The model under review builds one solid part; all positions refer to its coordinate system, in mm. A direction names the side the tool comes from. Coordinates: 2 decimals unless noted, no trailing zeros. Order: outer loops, then holes, each group sorted by start corner. A loop starts at its lowest first (then second) coordinate and runs counter-clockwise, first axis right, second up. Notation, with made-up numbers: M 55,54.25 L 67,54.25 A9 ccw 67,59.25 Z; hole C 34,80 d5. An arc over 180 degrees is marked long. One line per item, written item: value.
Autodesk Inventor part; units mm, degrees
ref_plane "YZ Plane" through (0, 0, 0) normal (1, 0, 0) x (0, 1, 0)
ref_plane "XZ Plane" through (0, 0, 0) normal (0, 1, 0) x (-1, 0, 0)
ref_plane "XY Plane" through (0, 0, 0) normal (0, 0, 1) x (1, 0, 0)
sketch "Sketch1" plane through (0, 0, 0) normal (0, 1, 0) x (-1, 0, 0)
  line L0 (4, -12.0702) -> (4, 30.9298)
  line L1 (4, 30.9298) -> (-1, 30.9298)
  line L2 (-1, 30.9298) -> (-1, 25.9298)
  line L3 (-1, 25.9298) -> (-22, 25.9298)
  line L4 (4, -12.0702) -> (-1, -12.0702)
  line L5 (-1, -12.0702) -> (-1, -12.0702)
  line L6 (-22, -8.0702) -> (-22, -8.0702)
  line L7 (-22, -8.0702) -> (-22, 3.3216)
  line L8 (-22, 3.3216) -> (-22, 3.3216)
  line L9 (-22, 3.3216) -> (-22, 25.9298)
  line L10 (-1, -12.0702) -> (-5, -12.0702)
  line L11 (-5, -12.0702) -> (-5, -9.0702)
  line L12 (-5, -9.0702) -> (-16, -9.0702)
  arc A0 (-22, -11.4735) -> (-16, -11.4735) centre (-19, -15.0915) ccw
  line L13 (-16, -9.0702) -> (-16, -11.4735)
  line L14 (-22, -8.0702) -> (-22, -11.4735)
  point P0 (0, 0)
  dimension "d28" = 5
  dimension "d30" = 0
  dimension "d69" = 5
  dimension "d118" = 4
  dimension "d119" = 3
  dimension "d130" = 4.7
  dimension "d148" = 35
  dimension "d151" = 2.4033
extrude "Extrusion1" add sketch "Sketch1" along normal blind 13
sketch "Sketch5" plane through (0, 13, 0) normal (0, 1, 0) x (1, 0, 0)
  line L0 (-4, -30.9298) -> (1, -30.9298)
  line L1 (-1, -30.9298) -> (-4, -30.9298)
  line L2 (-4, -30.9298) -> (-4, -25.9298)
  line L3 (-4, -25.9298) -> (-1, -25.9298)
  line L4 (-1, -25.9298) -> (-1, -30.9298)
  line L5 (1, -30.9298) -> (1, -25.9298)
  line L6 (-4, 1.8702) -> (-1, 1.8702)
  line L7 (-1, 1.8702) -> (-1, -3.1298)
  line L8 (-1, -3.1298) -> (-4, -3.1298)
  line L9 (-4, -3.1298) -> (-4, 1.8702)
  line L10 (1, 12.0702) -> (1, 17.0702)
  line L11 (5, 12.0702) -> (-4, 12.0702)
  point P0 (0, 0)
  point P1 (-4, 12.0702)
  dimension "d60" = 5
  dimension "d61" = 3
  dimension "d62" = 2
  dimension "d63" = 2
  dimension "d64" = 3
  dimension "d65" = 5
  dimension "d149" = 22.8
extrude "Extrusion6" add sketch "Sketch5" along normal blind 12.3
sketch "Sketch6" plane through (-1, 13, 30.9298) normal (1, 0, 0) x (0, 0, -1)
  circle A0 centre (2.5, 6.15) radius 1
  line L0 (0, 12.3) -> (5, 12.3)
  line L1 (0, 0) -> (0, 12.3)
  circle A1 centre (30.3, 6.15) radius 1
  line L2 (27.8, 12.3) -> (32.8, 12.3)
  line L3 (27.8, 0) -> (27.8, 12.3)
  point P0 (30.9298, -13)
  dimension "d70" = 2
  dimension "d71" = 6.15
  dimension "d72" = 2.5
  dimension "d73" = 2
  dimension "d74" = 6.15
  dimension "d75" = 2.5
extrude "Extrusion7" cut sketch "Sketch6" against normal blind 12.3
thread "Thread6"
thread "Thread7"
sketch "Sketch10" plane through (0, 13, 0) normal (0, 1, 0) x (1, 0, 0)
  circle A0 centre (0.6, 10.2702) radius 1
  circle A1 centre (19.4, 10.2702) radius 1
  circle A2 centre (10, -8.7298) radius 1
  line L0 (1, -25.9298) -> (22, -25.9298)
  line L1 (-4, -3.1298) -> (-4, -25.9298)
  line L2 (5, 12.0702) -> (-4, 12.0702)
  line L3 (5, 9.0702) -> (5, 12.0702)
  line L4 (5, 12.0702) -> (1, 12.0702)
  point P0 (0, 0)
  point P1 (1, 17.0702)
  point P2 (-1, 17.0702)
  point P3 (-4, 12.0702)
  dimension "d108" = 2
  dimension "d109" = 2
  dimension "d110" = 2
  dimension "d111" = 9.4
  dimension "d112" = 9.4
  dimension "d113" = 19
  dimension "d117" = 19
  dimension "d121" = 14
  dimension "d150" = 1.8
extrude "Extrusion11" cut sketch "Sketch10" against normal blind 15
sketch "Sketch13" plane through (0, 13, 0) normal (0, 1, 0) x (1, 0, 0)
  point P0 (0, 0)
sketch "Sketch14" plane through (0, 0, 0) normal (0, -1, 0) x (1, 0, 0)
  circle A0 centre (19.4611, -14.5702) radius 2
  circle A1 centre (19.4, -10.2702) radius 1
  point P0 (0, 0)
  dimension "d131" = 4
  dimension "d132" = 4.3
extrude "Extrusion12" cut sketch "Sketch14" against normal blind 6 contours A0
sketch "Sketch15" plane through (0, 13, 0) normal (0, 1, 0) x (1, 0, 0)
  arc A0 (22, 11.4735) -> (16, 11.4735) centre (19, 15.0915) ccw
  line L0 (15.3998, 12.0702) -> (22.6002, 12.0702)
  arc A1 (22.6002, 12.0702) -> (15.3998, 12.0702) centre (19, 15.0915) ccw
  line L1 (1, -25.9298) -> (22, -25.9298)
  point P0 (0, 0)
  dimension "d135" = 22.8
extrude "Extrusion13" add sketch "Sketch15" along normal blind 12.5
sketch "Sketch16" plane through (0, 25.5, 0) normal (0, 1, 0) x (1, 0, 0)
  arc A0 (22, 11.4735) -> (16, 11.4735) centre (19, 15.0915) ccw
  circle A1 centre (19, 15.0915) radius 5
  point P0 (0, 0)
  dimension "d138" = 10
extrude "Extrusion14" add sketch "Sketch16" along normal mid plane 25
sketch "Sketch18" plane through (19, 38, -15.0915) normal (0, 1, 0) x (1, 0, 0)
  circle A0 centre (0, 0) radius 5
  point P0 (-19, -15.0915)
extrude "Extrusion16" add sketch "Sketch18" along normal blind 12.5
sketch "Sketch19" plane through (19, 50.5, -15.0915) normal (0, 1, 0) x (1, 0, 0)
  circle A0 centre (0, 0) radius 1.9
  point P0 (-19, -15.0915)
  dimension "d154" = 3.8
extrude "Extrusion17" add sketch "Sketch19" along normal blind 5
properties part number "4_2.(new).stl"
(1) Tool access review of faces 1 (the flat face through (19, 50.5, -13)), 2 (the cylindrical face through (19.94, 6.59, -11.11)), 3 (the flat face through (1, 6, 28)), 4 (the flat face through (0, 6, -12.07)): name each direction out of +Z, -Z, +X, -X, +Y, -Y from which nothing blocks a thin tool from reaching the whole face with its end or side.
Geometry results:
face 1: +Y
face 2: -Y
face 3: +Z, +X, +Y, -Y
face 4: -Z, -X, +Y, -Y
(2) For L1, parallel to X at y = 8, z = -11; L2, parallel to Z at x = 19.4, y = 5.25; L3, parallel to Z at x = 0.6, y = 6.75, list the stretches that pass through material, from the lowest coordinate up.
Geometry results:
L1: x = -4 to -0.08, 1.28 to 5, 16 to 18.72, 20.08 to 22
L2: z = -19.77 to -16.57, -12.57 to -11.27, -9.27 to 25.93
L3: z = -12.07 to -11.27, -9.27 to 30.93
(3) We need section A-A, the plane x = 10. State the section outline as (y, z) points.
Geometry results:
outline: M 0,-9.07 L 13,-9.07 L 13,7.73 L 0,7.73 Z; M 0,9.73 L 13,9.73 L 13,25.93 L 0,25.93 Z
(4) Mouldability with a two-part tool opening along Z and no side actions: class faces 5 (the flat face through (-3, 19, 25.93)), 6 (the cylindrical face through (17.92, 32.01, -10.21)), 7 (the flat face through (-1, 19, 30)) as +Z half, -Z half, draft (parallel to the pull), parting line (faces both ways), or undercut.
Geometry results:
face 5: undercut
face 6: parting line
face 7: draft
(5) We need section B-B, the plane y = 19.15. State the section outline as (x, z) points, plus the area to 3 significant figures.
Geometry results:
outline: M -4,-1.87 L -1,-1.87 L -1,-0.37 L -4,-0.37 Z; M -4,1.63 L -1,1.63 L -1,3.13 L -4,3.13 Z; M -4,25.93 L -1,25.93 L -1,27.43 L -4,27.43 Z; M -4,29.43 L -1,29.43 L -1,30.93 L -4,30.93 Z; C 19,-15.09 d10
area: 96.5 mm2
(6) We need section D-D, the plane y = 7.5. State the section outline as (x, z) points, plus the area to 3 significant figures.
Geometry results:
outline: M -4,-12.07 L 5,-12.07 L 5,-9.07 L 16,-9.07 L 16,-11.47 A4.7 ccw long 22,-11.47 L 22,25.93 L 1,25.93 L 1,30.93 L -4,30.93 Z; hole C 0.6,-10.27 d2; hole C 10,8.73 d2; hole C 19.4,-10.27 d2
area: 1,030 mm2
(7) We need section C-C, the plane x = -2. State the section outline as (y, z) points.
Geometry results:
outline: M 0,-12.07 L 13,-12.07 L 13,-1.87 L 25.3,-1.87 L 25.3,3.13 L 13,3.13 L 13,25.93 L 25.3,25.93 L 25.3,30.93 L 0,30.93 Z; hole C 19.15,0.63 d2; hole C 19.15,28.43 d2
(8) Insertion check: pin 1 Ø1.2 at (x, z) = (20.5, -14.5) entering from -Y; pin 2 Ø5.5 at (x, y) = (10.5, 9) entering from -Z; pin 3 Ø1.5 at (x, y) = (-3, 17) entering from -Z. Each pin has a flat end and moves straight along its axis. Give the tip position at first contact, or say it passes through.
Geometry results:
pin 1: stops at y = 6
pin 2: stops at z = -9.07
pin 3: stops at z = -1.87
